```python
from build123d import *

# Parameters (mm, degrees)
SKETCH1_R           = 1.45
BOSS_EXTRUDE1_DEPTH = 2.4
FILLET1_R           = 0.5


with BuildPart() as part:
    # Sketch1 → Boss-Extrude1 (new body)
    with BuildSketch(Plane(origin=(0, 0, 0), x_dir=(1, 0, 0), z_dir=(0, 1, 0))):
        Polygon((0, 3.117691454), (-2.7, 1.558845727), (-2.7, -1.558845727), (0, -3.117691454), (2.7, -1.558845727), (2.7, 1.558845727), align=None)
        Circle(SKETCH1_R, mode=Mode.SUBTRACT)
    extrude(amount=BOSS_EXTRUDE1_DEPTH)

    # Fillet1
    fillet1_edges = [part.edges().sort_by_distance(p)[0] for p in [
        (2.7, 1.2, -1.558845727),
        (2.7, 1.2, 1.558845727),
        (0, 1.2, 3.117691454),
        (-2.7, 1.2, 1.558845727),
        (-2.7, 1.2, -1.558845727),
        (0, 1.2, -3.117691454),
        (-2.7, 2.4, 0),
        (-1.35, 2.4, 2.33826859),
        (1.35, 2.4, 2.33826859),
        (2.7, 2.4, 0),
        (1.35, 2.4, -2.33826859),
        (2.7, 0, 0),
        (1.35, 0, 2.33826859),
        (-1.35, 0, 2.33826859),
        (-2.7, 0, 0),
        (-1.35, 0, -2.33826859),
        (1.35, 0, -2.33826859),
        (-1.35, 2.4, -2.33826859),
    ]]
    fillet(fillet1_edges, radius=FILLET1_R)


solid = part.part
```
Design review of the part built by this model. Coordinates are the model's own, in mm. Give positions to 0.01 mm unless a question says otherwise; leave off trailing zeros. Order: outer loops, then holes, each group sorted by start corner. A loop starts at its lowest first (then second) coordinate and runs counter-clockwise, first axis right, second up. Notation, with made-up numbers: M 48.5,-19 L 103.5,-19 A19 cw 103.5,-2 Z; hole C -39,87 d5. An arc over 180 degrees is marked long. One line per question, with ' | ' between items. Start each with the question number.
Q1. We need section A-A (z = 1). Write out the cut boundary in (x, y), plus the area to 3 significant figures.
Q2. The part is to be moulded in two halves that separate along Z. For faces 1 (the face through (-1.45, 1.18, -0.06)), 2 (the face through (0, 2.4, 2)), 3 (the face through (1.263, 0.15, -2.224)), say which applies: +Z half, -Z half, draft (parallel to the pull), parting line (faces both ways), or undercut.
Q3. For L1, parallel to X at y = 1.85, z = 0; L2, parallel to Z at x = 0, y = 1.55; L3, parallel to Z at x = 1.15, y = 0.2, list the stretches that pass through material, from the lowest coordinate up. Write a range as [from, to].
Q4. We need section D-D (y = 0.4). Write out the cut boundary in (x, z), plus the area to 3 significant figures.
Q5. We need section C-C (z = 0). Write out the cut boundary in (x, y), plus the area to 3 significant figures.
Q6. We need section B-B (y = 1.7). Write out the cut boundary in (x, z).
Returned:
1) outline: M -2.7,0.5 A0.5 ccw -2.2,0 L -1.05,0 L -1.05,2.4 L -2.2,2.4 A0.5 ccw -2.7,1.9 Z; M 1.05,0 L 2.2,0 A0.5 ccw 2.7,0.5 L 2.7,1.9 A0.5 ccw 2.2,2.4 L 1.05,2.4 Z | area: 7.71 mm2
2) face 1: undercut | face 2: draft | face 3: -Z half
3) L1: [-2.7, -1.45], [1.45, 2.7] | L2: [-3.04, -1.45], [1.45, 3.04] | L3: [-2.34, -0.88], [0.88, 2.34]
4) outline: M -2.69,-1.27 A0.49 ccw -2.44,-1.69 L -0.24,-2.96 A0.49 ccw 0.24,-2.96 L 2.44,-1.69 A0.49 ccw 2.69,-1.27 L 2.69,1.27 A0.49 ccw 2.44,1.69 L 0.24,2.96 A0.49 ccw -0.24,2.96 L -2.44,1.69 A0.49 ccw -2.69,1.27 Z; hole C 0,0 d2.9 | area: 18.4 mm2
5) outline: M -2.7,0.5 A0.5 ccw -2.2,0 L -1.45,0 L -1.45,2.4 L -2.2,2.4 A0.5 ccw -2.7,1.9 Z; M 1.45,0 L 2.2,0 A0.5 ccw 2.7,0.5 L 2.7,1.9 A0.5 ccw 2.2,2.4 L 1.45,2.4 Z | area: 5.79 mm2
6) outline: M -2.7,-1.27 A0.5 ccw -2.45,-1.7 L -0.25,-2.97 A0.5 ccw 0.25,-2.97 L 2.45,-1.7 A0.5 ccw 2.7,-1.27 L 2.7,1.27 A0.5 ccw 2.45,1.7 L 0.25,2.97 A0.5 ccw -0.25,2.97 L -2.45,1.7 A0.5 ccw -2.7,1.27 Z; hole C 0,0 d2.9
